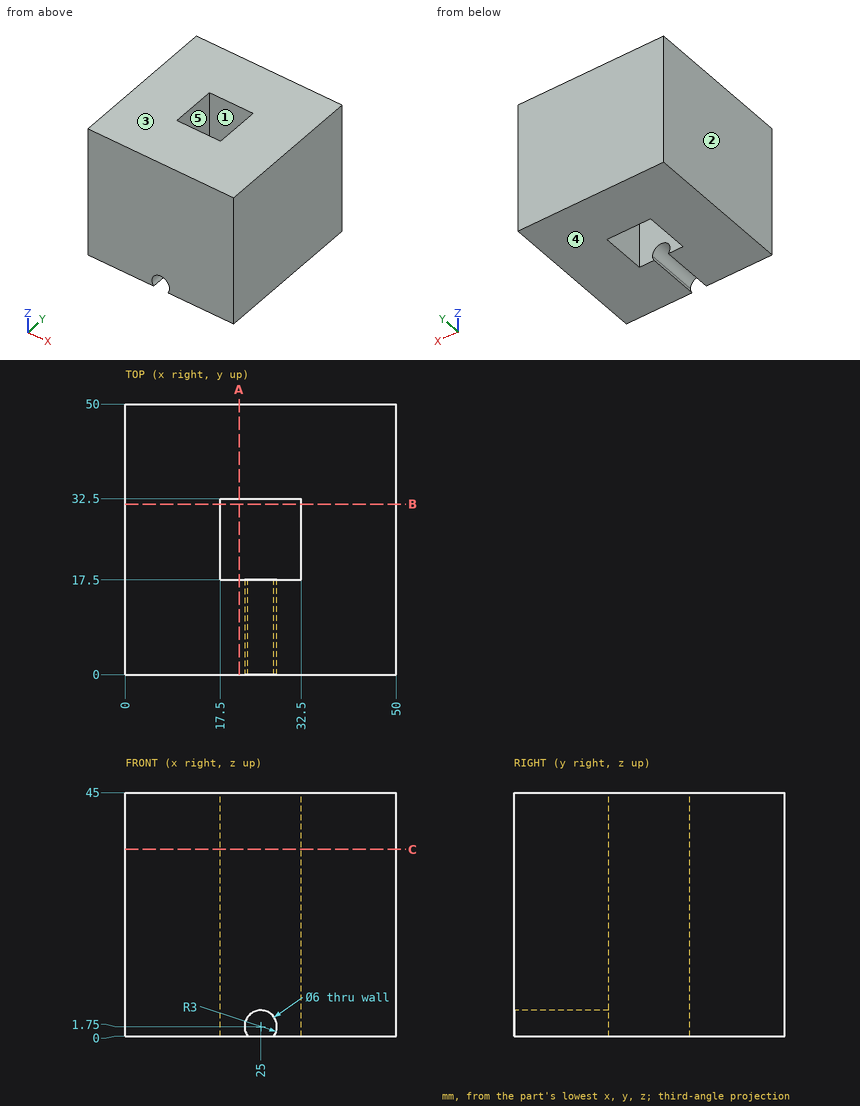
Geometry check sheet. Reference: drawing and pictorial views, mm from the part's lowest x, y, z. A direction names the side the tool comes from. Round coordinates to 2 decimals unless told otherwise and drop trailing zeros. Order: outer loops, then holes, each group sorted by start corner. A loop starts at its lowest first (then second) coordinate and runs counter-clockwise, first axis right, second up. Notation, with made-up numbers: (-25, 6) - (34, 6) arc R6 cw to (34, 11) - close; hole circle Ø2 at (56.25, 32.25). An arc over 180 degrees is marked (long way). One line per question, with ' | ' between items. Start each with the question number.
(1) Sectioned sample at C-C on z = 34.5. Record the cut outline in (x, y).
(2) Thickness scan on L1, parallel to X at y = 19, z = 16; L2, parallel to Z at x = 25, y = 6. Record the ranges inside material, lowest first. Write a range as [from, to].
(3) Access from +Z, -Z, +X, -X, +Y, -Y to the whole of each face (thin tool, end or side, straight path). Record for the marked faces 4 and 5.
(4) Sectioned sample at A-A on x = 21. Record the cut outline in (y, z).
(5) Release check for a two-part mould opening along X. For the marked faces 1, 2 and 3 record: released by +X, released by -X, zero draft, split by the parting line, or undercut.
Conclusion:
1) outline: (0, 0) - (50, 0) - (50, 50) - (0, 50) - close; hole (17.5, 17.5) - (32.5, 17.5) - (32.5, 32.5) - (17.5, 32.5) - close
2) L1: x = [0, 17.5], [32.5, 50] | L2: z = [4.75, 45]
3) face 4: -Z, +X, -X, +Y, -Y | face 5: +Z, -Z
4) outline: (0, 0) - (17.5, 0) - (17.5, 45) - (0, 45) - close; (32.5, 0) - (50, 0) - (50, 45) - (32.5, 45) - close
5) face 1: undercut | face 2: released by -X | face 3: zero draft
